from build123d import *

# Parameters (mm, degrees)
FILLET1_R           = 5
FILLET2_R           = 5
FILLET3_R           = 2
SKETCH3_W           = 10
SKETCH3_H           = 5
BOSS_EXTRUDE1_DEPTH = 25
BOSS_EXTRUDE2_REACH = 153.483
SKETCH4_W           = 10
SKETCH4_H           = 50


with BuildPart() as part:
    # Sketch1 → Revolve1 (revolve)
    with BuildSketch(Plane.XY, mode=Mode.PRIVATE) as revolve1_sk:
        Polygon((0, -50), (10, -50), (40, -30), (40, 0), (20, 0), (20, -25), (0, -25), align=None)
    revolve(revolve1_sk.sketch.rotate(Axis((-91.89476197, 0, 0), (1, 0, 0)), 270), axis=Axis((-91.89476197, 0, 0), (1, 0, 0)))

    # Sketch2 → Revolve3 (revolve)
    with BuildSketch(Plane.XY):
        with BuildLine():
            Line((40, -20), (60, -20))
            Line((60, -20), (100, -2))
            ThreePointArc((100, -2), (101.414213562, -1.414213562), (102, 0))
            Line((102, 0), (100, 0))
            Line((100, 0), (40, 0))
            Line((40, 0), (40, -20))
        make_face()
    revolve(axis=Axis((100, 0, 0), (-1, 0, 0)))

    # Fillet1
    fillet1_edges = [part.edges().sort_by_distance(p)[0] for p in [
        (40, 20, 0),
        (60, 20, 0),
        (40, 0, -30),
        (10, 0, -50),
        (0, 0, -50),
    ]]
    fillet(fillet1_edges, radius=FILLET1_R)

    # Fillet2
    fillet2_edges = [part.edges().sort_by_distance(p)[0] for p in [
        (100, 2, 0),
    ]]
    fillet(fillet2_edges, radius=FILLET2_R)

    # Fillet3
    fillet3_edges = [part.edges().sort_by_distance(p)[0] for p in [
        (0, 0, -25),
    ]]
    fillet(fillet3_edges, radius=FILLET3_R)

    # Sketch4 → Boss-Extrude2 (add, up to next)
    with BuildSketch(Plane(origin=(0, -50.215600765, 0), x_dir=(1, 0, 0), z_dir=(0, 1, 0)), mode=Mode.PRIVATE) as boss_extrude2_sk1:
        with Locations((10, 0)):
            Rectangle(SKETCH4_W, SKETCH4_H)
    boss_extrude2_tool1 = extrude(boss_extrude2_sk1.sketch, amount=BOSS_EXTRUDE2_REACH, mode=Mode.PRIVATE) - part.part


with BuildPart() as body_2:
    # Sketch3 → Boss-Extrude1 (new, symmetric)
    with BuildSketch(Plane.XY):
        with Locations((10, -52.715600765)):
            Rectangle(SKETCH3_W, SKETCH3_H)
    extrude(amount=BOSS_EXTRUDE1_DEPTH, both=True)


with BuildPart() as part_1:
    add(part.part)

    add(body_2.part)  # Boss-Extrude2 merges body 2
    add(boss_extrude2_tool1.solids().sort_by_distance((10, -50.215601, 0))[0])


solid = part_1.part
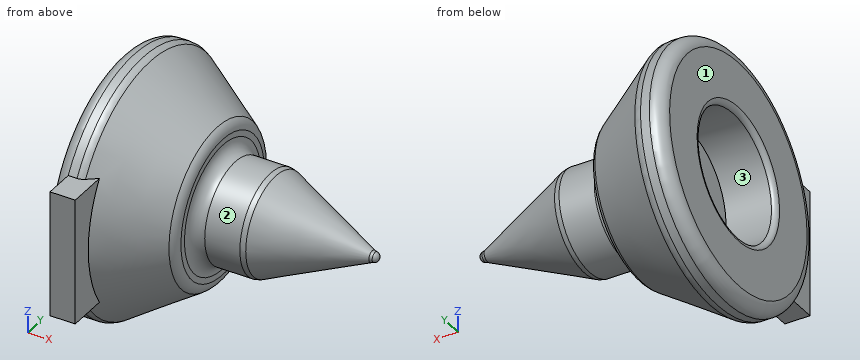
Geometry check sheet. Reference: the model listing, model coordinates, mm. Face numbers are marked on the shaded views. A direction names the side the tool comes from. Give positions to 0.01 mm unless a question says otherwise; leave off trailing zeros. Order: outer loops, then holes, each group sorted by start corner. A loop starts at its lowest first (then second) coordinate and runs counter-clockwise, first axis right, second up. Notation, with made-up numbers: (20, 61) - (36, 61) arc R12 ccw to (36, 71) - close; hole circle Ø4 at (-2, 43). An arc over 180 degrees is marked (long way). Use one line per item in the form item = value.
1) Material ranges on probe 1 along Y at (x, z) = (6, 0); probe 2 along X at (y, z) = (-47, 24); probe 3 along Y at (x, z) = (14.5, 0), recorded low to high. Write a range as from..to.
Working result:
probe_1 = -55.22..-25, 25..50
probe_2 = 5..15
probe_3 = -55.22..-25, 25..47
2) Sectioned sample at C-C (x = 25.5). Record the boundary of the cut face in (y, z), and give its area (3 significant figures).
Working result:
outline = circle Ø79.33 at (0, 0)
area = 4,940 mm^2
3) Depth check by flat-ended pin: pin 1 Ø10 at (x, z) = (39.5, -20) entering from -Y; pin 2 Ø5 at (x, y) = (8.5, -45.5) entering from -Z; pin 3 Ø1 at (y, z) = (-0.5, -6.5) entering from +X. Enter the tip coordinate at first touch or a pass-through.
Working result:
pin_1 = -28.28
pin_2 = -25.51
pin_3 = 91.07
4) Sectioned sample at A-A (x = 7). Record the boundary of the cut face in (y, z), and give its area (3 significant figures).
Working result:
outline = (-55.22, -25) - (-43.3, -25) arc R50 ccw (long way) to (-43.3, 25) - (-55.22, 25) - close; hole circle Ø50 at (0, 0)
area = 6,260 mm^2
5) Access from +Z, -Z, +X, -X, +Y, -Y to the whole of each face (thin tool, end or side, straight path). Record for the marked faces 1, 2 and 3.
Working result:
face_1 = +Z, -Z, -X, +Y, -Y
face_2 = +X
face_3 = -X
6) Sectioned sample at B-B (x = 69). Record the boundary of the cut face in (y, z).
Working result:
outline = circle Ø31.9 at (0, 0)
